from build123d import *

# Parameters (mm, degrees)
F0_R     = 40
F0_R_2   = 7.5
F1_DEPTH = 2
F2_DEPTH = 10
F3_R     = 9
F3_R_2   = 7.5
F4_DEPTH = 1.5
F5_SIZE  = 1.49999


# Not quite as in the source:
# - a fillet or chamfer is up to 0.001 mm smaller than in the source, because OpenCascade refuses the exact size


with BuildPart() as f1:
    # F0 (on Top) → F1 (new body)
    with BuildSketch(Plane.XY):
        Circle(F0_R)
        with Locations((0, -30)):
            Circle(F0_R_2, mode=Mode.SUBTRACT)
        with Locations((-30, 0)):
            Circle(F0_R_2, mode=Mode.SUBTRACT)
        with Locations((30, 0)):
            Circle(F0_R_2, mode=Mode.SUBTRACT)
        with BuildLine():
            ThreePointArc((0, 22.5), (-5.3033008589, 35.3033008589), (7.5, 30))
            ThreePointArc((7.5, 30), (5.3033008589, 24.6966991411), (0, 22.5))
        make_face(mode=Mode.SUBTRACT)
    extrude(amount=F1_DEPTH)

    # F0 (on Top) → F2 (join)
    with BuildSketch(Plane.XY):
        with Locations((0, -30)):
            Circle(F0_R_2)
        with Locations((30, 0)):
            Circle(F0_R_2)
        with BuildLine():
            ThreePointArc((0, 22.5), (5.3033008589, 24.6966991411), (7.5, 30))
            ThreePointArc((7.5, 30), (-5.3033008589, 35.3033008589), (0, 22.5))
        make_face()
        with Locations((-30, 0)):
            Circle(F0_R_2)
    extrude(amount=F2_DEPTH)

    # F3 (on face) → F4 (join)
    with BuildSketch(Plane.XY.offset(10)):
        with Locations((-30, 0)):
            Circle(F3_R)
        with Locations((0, -30)):
            Circle(F3_R)
        with Locations((0, -30)):
            Circle(F3_R_2, mode=Mode.SUBTRACT)
        with Locations((0, -30)):
            Circle(F3_R_2)
        with Locations((30, 0)):
            Circle(F3_R)
        with Locations((0, 30)):
            Circle(F3_R)
    extrude(amount=F4_DEPTH)

    # F5 (size 1.5 in the source; OpenCascade refuses exactly that, so slightly less here)
    f5_edges = [f1.edges().sort_by_distance(p)[0] for p in [
        (-9, 30, 10),
        (-39, 0, 10),
        (-9, -30, 10),
        (21, 0, 10),
    ]]
    chamfer(f5_edges, length=F5_SIZE)


solid = f1.part
Could you check a few things on this model? Use its own coordinates, in mm. A direction names the side the tool comes from. Coordinates: 2 decimals unless noted, no trailing zeros. Write each loop counter-clockwise with the first axis right and the second up, starting at its lowest first coordinate (ties: lowest second). Pieces come first, ordered by that corner, then holes. Notation, with made-up numbers: (71, 54.5) - (109, 54.5) arc R22 ccw to (109, 79.5) - close; hole circle Ø7 at (20, 25.5). An arc over 180 degrees is marked (long way). Put each result on its own line as item: value. Start each with the question number.
Q1. Which directions (+Z, -Z, +X, -X, +Y, -Y) give clear straight access to the entire face, cutting with the end or side of a thin tool? Please do faces 1 (the flat face through (0, -30, 11.5)), 2 (the cylindrical face through (7.154, 32.253, 5.944)).
Q2. Please list where these lines run through material, in increasing order: L1, parallel to X at y = -6, z = 7.75; L2, parallel to Z at x = 7, y = 9; L3, parallel to X at y = -5.5, z = 3.
Q3. Thinking about a two-plate mould opening in Y: for faces 3 (the cylindrical face through (-1.63, -37.32, 5.94)), 4 (the cylindrical face through (-8.67, -39.05, 0.99)), 5 (the flat face through (-30, 0, 11.5)), which applies, pulls with the +Y half, pulls with the -Y half, needs draft (parallel to the pull), parting line crosses it, or undercut?
Q4. I'm going to push flat-ended pins straight in: P1, Ø1, axis at y = -27, z = 8.5, coming from the +X side; P2, Ø1.5, axis at x = -0.5, y = -6, coming from the +Z side; P3, Ø3, axis at x = -24.5, z = 7.5, coming from the -Y side. Where does each tip first touch, or does it pass through?
Q5. I want a section at B-B on z = 6.25. Write out the boundary of the cut face in (x, y).
Checks:
1. face 1: +Z, +X, -X, +Y, -Y
1. face 2: none
2. L1: -34.5 to -25.5, 25.5 to 34.5
2. L2: 0 to 2
2. L3: -35.1 to -24.9, 24.9 to 35.1
3. face 3: undercut
3. face 4: parting line crosses it
3. face 5: needs draft
4. P1: x = 7.07
4. P2: z = 2
4. P3: y = -6.34
5. outline: circle Ø15 at (-30, 0); circle Ø15 at (0, -30); circle Ø15 at (0, 30); circle Ø15 at (30, 0)
